Geometry: final body of the model. Coordinates: model frame, mm. A direction names the side the tool comes from. Coordinates: 2 decimals unless noted, no trailing zeros. Order: outer loops, then holes, each group sorted by start corner. A loop starts at its lowest first (then second) coordinate and runs counter-clockwise, first axis right, second up. Notation, with made-up numbers: M 39,-26 L 59,-26 A25 ccw 59,-7 Z; hole C -16.75,31 d6. An arc over 180 degrees is marked long. Write item = value, one per line.
from build123d import *

# Parameters (mm, degrees)
SKETCH_1_W          = 200
SKETCH_1_H          = 270
EXTRUDE_1_DEPTH     = 200
SHELL_1_T           = -2
SKETCH_2_R          = 3.5
CUT_EXTRUDE_1_DEPTH = 10


with BuildPart() as part:
    # 草图1 → 凸台-拉伸1 (new body)
    with BuildSketch(Plane(origin=(0, 0, 0), x_dir=(1, 0, 0), z_dir=(0, 1, 0))):
        Rectangle(SKETCH_1_W, SKETCH_1_H)
    extrude(amount=EXTRUDE_1_DEPTH)

    # 抽壳1
    shell_1_openings = [part.faces().sort_by_distance(p)[0] for p in [
        (0, 200, 0),
    ]]
    offset(amount=SHELL_1_T, openings=shell_1_openings, kind=Kind.INTERSECTION)

    # 草图2 → 切除-拉伸1 (cut)
    with BuildSketch(Plane(origin=(0, 0, 0), x_dir=(-1, 0, 0), z_dir=(0, -1, 0))):
        with Locations(Location((90, -125, 0), (0, 0, 90))):
            Circle(SKETCH_2_R)
        with Locations(Location((-90, -125, 0), (0, 0, 90))):
            Circle(SKETCH_2_R)
        with Locations(Location((-90, 125, 0), (0, 0, 90))):
            Circle(SKETCH_2_R)
        with Locations(Location((90, 125, 0), (0, 0, 90))):
            Circle(SKETCH_2_R)
    extrude(amount=-CUT_EXTRUDE_1_DEPTH, mode=Mode.SUBTRACT)


solid = part.part
1) Section B-B, the plane z = 125. Return loops of the section in (x, y), and give its area (3 significant figures).
Numbers:
outline = M -100,0 L -93.5,0 L -93.5,2 L -98,2 L -98,200 L -100,200 Z; M -86.5,0 L 86.5,0 L 86.5,2 L -86.5,2 Z; M 93.5,0 L 100,0 L 100,200 L 98,200 L 98,2 L 93.5,2 Z
area = 1,160 mm²
2) Section C-C, the plane y = 122.5. Return loops of the section in (x, z).
Numbers:
outline = M -100,-135 L 100,-135 L 100,135 L -100,135 Z; hole M -98,-133 L 98,-133 L 98,133 L -98,133 Z
3) Set-up query: faces 1 (the face through (-1, 100, -133)), 2 (the face through (88.659, 0.986, -128.233)). Return all of +Z, -Z, +X, -X, +Y, -Y with unobstructed straight access to the full face (end or side cutting, diameter ignored); none if empty.
Numbers:
face_1 = +Y
face_2 = +Y, -Y
4) Pin query (flat end, axial travel): pin 1 (9 mm diameter, centred on x = 90, z = 125, fed in from +Y); pin 2 (8 mm diameter, centred on x = 55.5, z = -8, fed in from -Y). Return the tip coordinate at first contact, or that it passes through.
Numbers:
pin_1 = 2
pin_2 = 0
5) Mould query, pull axis Z, two halves, no side actions, for faces 3 (the face through (-1, 99, -135)), 4 (the face through (-98, 100, 2)), 5 (the face through (-1, 100, 133)), 6 (the face through (-100, 99, 2)). Classes: pulls with the +Z half, pulls with the -Z half, needs draft (parallel to the pull), parting line crosses it, or undercut.
Numbers:
face_3 = pulls with the -Z half
face_4 = undercut
face_5 = undercut
face_6 = needs draft
6) Section D-D, the plane x = -12.5. Return loops of the section in (y, z), and give its area (3 significant figures).
Numbers:
outline = M 0,-135 L 200,-135 L 200,-133 L 2,-133 L 2,133 L 200,133 L 200,135 L 0,135 Z
area = 1,330 mm²
7) Section A-A, the plane x = -90. Return loops of the section in (y, z).
Numbers:
outline = M 0,-135 L 200,-135 L 200,-133 L 2,-133 L 2,-128.5 L 0,-128.5 Z; M 0,-121.5 L 2,-121.5 L 2,121.5 L 0,121.5 Z; M 0,128.5 L 2,128.5 L 2,133 L 200,133 L 200,135 L 0,135 Z
8) Line query: L1, parallel to X at y = 1, z = -125; L2, parallel to X at y = 112.5, z = 14.5; L3, parallel to Z at x = -75, y = 95.5. Output: solid intervals per line, ascending.
Numbers:
L1 = -100 to -93.5, -86.5 to 86.5, 93.5 to 100
L2 = -100 to -98, 98 to 100
L3 = -135 to -133, 133 to 135
